Design review of the part built by this model. Coordinates are the model's own, in mm. Face numbers are marked on the shaded views. A direction names the side the tool comes from. Coordinates: 2 decimals unless noted, no trailing zeros. Write each loop counter-clockwise with the first axis right and the second up, starting at its lowest first coordinate (ties: lowest second). Pieces come first, ordered by that corner, then holes.
Q1. For pin 1 Ø4 at (x, z) = (-9.5, 93) entering from -Y; pin 2 Ø20 at (x, z) = (2.5, 132.5) entering from -Y; pin 3 Ø3 at (x, z) = (0, 16.5) entering from -Y, all flat-tipped, find the tip position at first contact; note any pin that passes through.
Q2. The part is to be moulded in two halves that separate along X. For the marked faces 1, 2 and 3, say which applies: released by +X, released by -X, zero draft, split by the parting line, or undercut.
Q3. Take a section at B-B, the plane z = 38. Write out the cut boundary in (x, y).
Q4. For the marked faces 4 and 5, list the 3-axis set-ups (+Z, -Z, +X, -X, +Y, -Y) from which the entire face can be reached by the end or side of a thin tool; tool diameter is ignored.
Q5. Take a section at A-A, the plane z = 125. Write out the cut boundary in (x, y).
Q6. For L1, parallel to Z at x = -14, y = 3.75; L2, parallel to Z at x = -14, y = 10.75 (3 decimals); L3, parallel to X at y = 11, z = 41.5 (3 decimals), list the stretches that pass through material, from the lowest coordinate up.
Q7. Take a section at C-C, the plane x = 2. Write out the cut boundary in (y, z).
Q8. Take a section at D-D, the plane z = 5. Write out the cut boundary in (x, y).
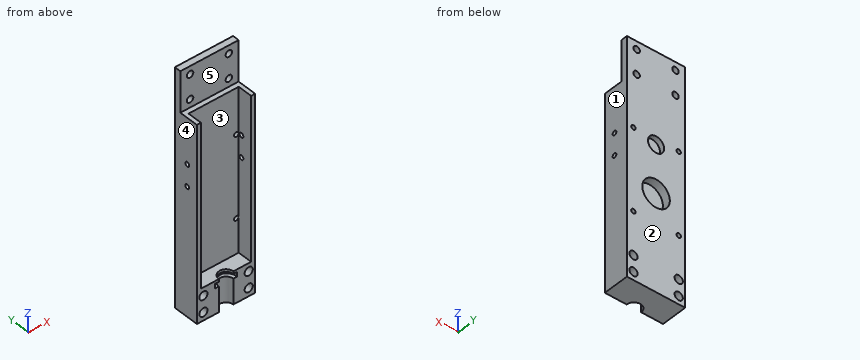
Autodesk Fusion 360 part; units mm, degrees
sketch "スケッチ1" plane through (0, 0, 0) normal (0, 0, 1) x (1, 0, 0)
  line L0 (-17.5, 11) -> (17.5, 11)
  line L1 (17.5, 11) -> (17.5, 0)
  line L2 (17.5, 0) -> (-17.5, 0)
  line L3 (-17.5, 0) -> (-17.5, 11)
  dimension "d1" = 35
  dimension "d2" = 11
extrude "押し出し1" add sketch "スケッチ1" along normal blind 120
sketch "スケッチ2" plane through (0, 0, 0) normal (0, 0, -1) x (1, 0, 0)
  line L0 (17.5, 0) -> (-17.5, 0)
  line L1 (-17.5, 0) -> (-17.5, -11)
  line L2 (-17.5, -11) -> (17.5, -11)
  line L3 (17.5, -11) -> (17.5, 0)
  circle A0 centre (0, 0) radius 4.5
  dimension "d5" = 9
extrude "押し出し2" cut sketch "スケッチ2" against normal blind 20 contours L0 A0 picked at (-0.548, -1.3963)
sketch "スケッチ3" plane through (0, 0, 120) normal (0, 0, 1) x (-1, 0, 0)
  line L0 (17.5, 0) -> (-17.5, 0)
  line L1 (-17.5, 0) -> (-17.5, -11)
  line L2 (-17.5, -11) -> (17.5, -11)
  line L3 (17.5, -11) -> (17.5, 0)
  line L4 (15.5, -9) -> (-15.5, -9)
  line L5 (-15.5, -9) -> (-15.5, 0)
  line L6 (-15.5, 0) -> (15.5, 0)
  line L7 (15.5, 0) -> (15.5, -9)
  dimension "d8" = 2
  dimension "d9" = 31
extrude "押し出し3" cut sketch "スケッチ3" against normal blind 100 contours L0 L4 L5 L6 L7
ref_plane "作業平面1" through (0, 5.5, 9) normal (0, 0, -1) x (-1, 0, 0)
sketch "スケッチ5" plane through (0, 11, 0) normal (0, 1, 0) x (-1, 0, 0)
  line L0 (-17.5, 0) -> (17.5, 0)
  line L1 (17.5, 0) -> (17.5, 120)
  line L2 (17.5, 120) -> (-17.5, 120)
  line L3 (-17.5, 120) -> (-17.5, 0)
  line L4 (-17.5, 130) -> (17.5, 130)
  line L5 (17.5, 130) -> (17.5, 120)
  line L6 (17.5, 120) -> (-17.5, 120)
  line L7 (-17.5, 120) -> (-17.5, 130)
  line L8 (-17.5, 125) -> (17.5, 125) construction
  circle A0 centre (12, 125) radius 2
  circle A1 centre (-12, 125) radius 2
  dimension "d16" = 4
  dimension "d17" = 4
  dimension "d18" = 24
  dimension "d19" = 10
  dimension "d20" = 5.5
extrude "押し出し5" add sketch "スケッチ5" against normal blind 2 contours L2 L4 L5 L6 L7
sketch "スケッチ8" plane through (0, 0, 0) normal (0, -1, 0) x (1, 0, 0)
  line L0 (-4.5, 20) -> (-15.5, 20)
  line L1 (-15.5, 20) -> (-15.5, 120)
  line L2 (-15.5, 120) -> (-17.5, 120)
  line L3 (-17.5, 120) -> (-17.5, 0)
  line L4 (-17.5, 0) -> (-4.5, 0)
  line L5 (-4.5, 0) -> (-4.5, 20)
  circle A0 centre (-14, 15) radius 2.55
  line L6 (18.5, 15) -> (-17.5, 15) construction
  line L7 (17.541, 5) -> (-17.5, 5) construction
  line L8 (15.5, 20) -> (4.5, 20) construction
  circle A1 centre (14, 15) radius 2.55
  circle A2 centre (14, 5) radius 2.55
  circle A3 centre (-14, 5) radius 2.55
  line L9 (17.5, 0) -> (17.5, 120)
  dimension "d30" = 5
  dimension "d31" = 10
  dimension "d32" = 5.1
  dimension "d33" = 5.1
  dimension "d34" = 5.1
  dimension "d35" = 5.1
  dimension "d36" = 3.5
  dimension "d37" = 3.5
  dimension "d38" = 3.5
  dimension "d39" = 3.5
extrude "押し出し8" cut sketch "スケッチ8" against normal blind 15 contours A0 | A1 | A2 | A3
move_face "OffsetFaces1" offset 3 1 faces at (-3.8517, 11, 52.6741)
sketch "Sketch9" plane through (0, 9, 0) normal (0, -1, 0) x (1, 0, 0)
  circle A0 centre (12, 125) radius 2
  circle A1 centre (-12, 125) radius 2
  line L0 (-15.5, 120) -> (-15.5, 20)
  line L1 (-15.5, 20) -> (15.5, 20)
  line L2 (15.5, 20) -> (15.5, 120)
  line L3 (15.5, 120) -> (17.5, 120)
  line L4 (17.5, 120) -> (17.5, 130)
  line L5 (17.5, 130) -> (-17.5, 130)
  line L6 (-17.5, 130) -> (-17.5, 120)
  line L7 (-17.5, 120) -> (-15.5, 120)
  point P0 (14, 41.5)
  point P1 (-14, 41.5)
  point P2 (-14, 92)
  point P3 (14, 92)
hole "Hole1" at (-14, 9, 92) at (14, 9, 92) at (14, 9, 41.5) at (-14, 9, 41.5) direction (0, 1, 0) diameter 2.75 depth 9 tip angle 118
ref_plane "WorkPlane2" through (0, 0, 17) normal (0, 0, 1) x (1, 0, 0)
sketch "Sketch13" plane through (0, 0, 17) normal (0, 0, 1) x (1, 0, 0)
  line L0 (3.3178, 6.05) -> (-3.3178, 6.05)
  arc A0 (-3.3178, 6.05) -> (3.3178, 6.05) centre (0, 0) ccw
  dimension "d63" = 13.8
extrude "Extrude9" cut sketch "Sketch13" along normal blind 1.4 and the other way blind 1.4
sketch "Sketch11" plane through (0, 9, 0) normal (0, -1, 0) x (1, 0, 0)
  circle A0 centre (-12, 125) radius 2
  circle A1 centre (12, 125) radius 2
  line L0 (-15.5, 120) -> (-15.5, 20)
  line L1 (-15.5, 20) -> (15.5, 20)
  line L2 (15.5, 20) -> (15.5, 120)
  line L3 (15.5, 120) -> (17.5, 120)
  line L4 (17.5, 120) -> (17.5, 130)
  line L5 (17.5, 130) -> (-17.5, 130)
  line L6 (-17.5, 130) -> (-17.5, 120)
  line L7 (-17.5, 120) -> (-15.5, 120)
  line L8 (-17.5, 130) -> (17.5, 130)
  line L9 (17.5, 130) -> (17.5, 120)
  line L10 (17.5, 120) -> (-17.5, 120)
  line L11 (-17.5, 120) -> (-17.5, 130)
  circle A2 centre (14, 41.5) radius 1.375
  circle A3 centre (-14, 92) radius 1.375
  circle A4 centre (14, 92) radius 1.375
  circle A5 centre (-14, 41.5) radius 1.375
extrude "Extrude10" cut sketch "Sketch11" against normal blind 3 contours L3 L4 L5 L6 L7 L8 L9 L10 L11
move_face "OffsetFaces2" offset 2 1 faces at (4.4189, 14, 58.7625)
move_face "OffsetFaces3" offset 15 1 faces at (5.8333, 13.3333, 130)
sketch "Sketch12" plane through (0, 12, 0) normal (0, -1, 0) x (1, 0, 0)
  circle A0 centre (12, 125) radius 2
  circle A1 centre (-12, 125) radius 2
  line L0 (-17.5, 120) -> (17.5, 120)
  line L1 (17.5, 120) -> (17.5, 145)
  line L2 (17.5, 145) -> (-17.5, 145)
  line L3 (-17.5, 145) -> (-17.5, 120)
  point P0 (-12, 140)
  point P1 (12, 140)
hole "Hole2" at (-12, 12, 140) at (12, 12, 140) direction (0, 1, 0) diameter 4 depth 5 tip angle 118
sketch "Sketch14" plane through (17.5, 0, 0) normal (1, 0, 0) x (0, 1, 0)
  line L0 (12, 120) -> (0, 120)
  line L1 (0, 120) -> (0, 0)
  line L2 (0, 0) -> (16, 0)
  line L3 (16, 0) -> (16, 145)
  line L4 (16, 145) -> (12, 145)
  line L5 (12, 145) -> (12, 120)
  line L6 (12, 120) -> (0, 120)
  line L7 (0, 120) -> (0, 0)
  line L8 (0, 0) -> (16, 0)
  line L9 (16, 0) -> (16, 145)
  line L10 (16, 145) -> (12, 145)
  line L11 (12, 145) -> (12, 120)
  point P0 (7, 92)
  point P1 (7, 78.5)
hole "Hole3" at (17.5, 7, 92) at (17.5, 7, 78.5) direction (-1, 0, 0) diameter 2.75 depth 200 tip angle 118
move_face "OffsetFaces4" offset 0.5 1 faces at (17.5, 7.6667, 25.7083)
move_face "OffsetFaces5" offset 0.5 1 faces at (-17.5, 7.6667, 25.7083)
sketch "Sketch15" plane through (0, 16, 0) normal (0, 1, 0) x (-1, 0, 0)
  circle A0 centre (12, 140) radius 2
  circle A1 centre (-12, 140) radius 2
  circle A2 centre (-14, 41.5) radius 1.375
  circle A3 centre (14, 92) radius 1.375
  circle A4 centre (-14, 92) radius 1.375
  circle A5 centre (14, 41.5) radius 1.375
  circle A6 centre (-14, 5) radius 2.55
  circle A7 centre (14, 5) radius 2.55
  circle A8 centre (-14, 15) radius 2.55
  circle A9 centre (14, 15) radius 2.55
  circle A10 centre (-12, 125) radius 2
  circle A11 centre (12, 125) radius 2
  line L0 (-18, 0) -> (18, 0)
  line L1 (18, 0) -> (18, 145)
  line L2 (18, 145) -> (-18, 145)
  line L3 (-18, 145) -> (-18, 0)
  point P0 (0, 89)
hole "Hole4" at (0, 16, 89) direction (0, -1, 0) diameter 10 depth 3 tip angle 180
sketch "Sketch17" plane through (0, 16, 0) normal (0, 1, 0) x (-1, 0, 0)
  point P0 (0, 59.5)
hole "Hole5" at (0, 16, 59.5) direction (0, -1, 0) diameter 17 depth 5 tip angle 180
Responses:
1. pin 1: stops at y = 9
1. pin 2: stops at y = 12
1. pin 3: stops at y = 4.34
2. face 1: released by +X
2. face 2: zero draft
2. face 3: undercut
3. outline: (-18, 0) - (-15.5, 0) - (-15.5, 9) - (15.5, 9) - (15.5, 0) - (18, 0) - (18, 16) - (-18, 16) - close
4. face 4: +Z, -Z, -X, +Y, -Y
4. face 5: +Z, +X, -X, -Y
5. outline: (-18, 12) - (-14, 12) - (-14, 16) - (-18, 16) - close; (-10, 12) - (10, 12) - (10, 16) - (-10, 16) - close; (14, 12) - (18, 12) - (18, 16) - (14, 16) - close
6. L1: z = 0 to 2.45, 7.55 to 12.45, 17.55 to 20
6. L2: z = 0 to 2.45, 7.55 to 12.45, 17.55 to 40.125, 42.875 to 90.625, 93.375 to 120
6. L3: x = -18 to -15.375, -12.625 to 12.625, 15.375 to 18
7. outline: (4.03, 0) - (16, 0) - (16, 51.24) - (11, 51.24) - (11, 67.76) - (16, 67.76) - (16, 84.42) - (13, 84.42) - (13, 93.58) - (16, 93.58) - (16, 145) - (12, 145) - (12, 120) - (9, 120) - (9, 20) - (4.03, 20) - (4.03, 18.4) - (6.05, 18.4) - (6.05, 15.6) - (4.03, 15.6) - close
8. outline: (-18, 0) - (-16.55, 0) - (-16.55, 16) - (-18, 16) - close; (-11.45, 0) - (-4.5, 0) arc R4.5 cw to (4.5, 0) - (11.45, 0) - (11.45, 16) - (-11.45, 16) - close; (16.55, 0) - (18, 0) - (18, 16) - (16.55, 16) - close
